```python
from build123d import *

# Parameters (mm, degrees)
SKETCH1_W              = 116
SKETCH1_H              = 60
SKETCH1_R              = 2
BOSS_EXTRUDE1_DEPTH    = 3
SKETCH2_R              = 1.75
ODROID_HOLES_DEPTH     = 4
CUT_EXTRUDE2_DEPTH     = 0.2
SKETCH4_R              = 1.75
PIXHAWK_PM_DEPTH       = 4
SKETCH5_R              = 1.75
BUCKCONVERTER_5A_DEPTH = 4
SKETCH6_R              = 2.5
SKETCH6_R_2            = 4.5
CUT_EXTRUDE5_DEPTH     = 4
FILLET1_R              = 5


with BuildPart() as part:
    # Sketch1 → Boss-Extrude1 (new body)
    with BuildSketch(Plane(origin=(0, 0, 0), x_dir=(1, 0, 0), z_dir=(0, 1, 0))):
        Rectangle(SKETCH1_W, SKETCH1_H)
        with Locations((53, 13)):
            Circle(SKETCH1_R, mode=Mode.SUBTRACT)
        with Locations((53, -13)):
            Circle(SKETCH1_R, mode=Mode.SUBTRACT)
        with Locations((-53, -13)):
            Circle(SKETCH1_R, mode=Mode.SUBTRACT)
        with Locations((-53, 13)):
            Circle(SKETCH1_R, mode=Mode.SUBTRACT)
    extrude(amount=BOSS_EXTRUDE1_DEPTH)

    # Sketch2 → Odroid-holes (cut, through all)
    with BuildSketch(Plane(origin=(0, 3, 0), x_dir=(1, 0, 0), z_dir=(0, 1, 0))):
        with Locations((38, 26)):
            Circle(SKETCH2_R)
        with Locations((38, -26)):
            Circle(SKETCH2_R)
        with Locations((-38, -26)):
            Circle(SKETCH2_R)
        with Locations((-38, 26)):
            Circle(SKETCH2_R)
    extrude(amount=-ODROID_HOLES_DEPTH, mode=Mode.SUBTRACT)

    # Sketch3 → Cut-Extrude2 (cut)
    with BuildSketch(Plane(origin=(0, 3, 0), x_dir=(1, 0, 0), z_dir=(0, 1, 0))):
        Polygon((-49.756039442, -1.122419343), (-49.756039442, -1.666214416), (-51.913411237, -0.552547549), (-51.913411237, -0.104155121), (-49.756039442, 1.009511746), (-49.756039442, 0.465080657), (-51.293930067, -0.328669343), align=None)
        Polygon((-47.110206109, -1.122419343), (-47.110206109, -1.666214416), (-49.267577904, -0.552547549), (-49.267577904, -0.104155121), (-47.110206109, 1.009511746), (-47.110206109, 0.465080657), (-48.648096734, -0.328669343), align=None)
        Polygon((-44.464372776, -1.122419343), (-44.464372776, -1.666214416), (-46.621744571, -0.552547549), (-46.621744571, -0.104155121), (-44.464372776, 1.009511746), (-44.464372776, 0.465080657), (-46.002263401, -0.328669343), align=None)
    extrude(amount=-CUT_EXTRUDE2_DEPTH, mode=Mode.SUBTRACT)

    # Sketch4 → Pixhawk-PM (cut, through all)
    with BuildSketch(Plane(origin=(0, 3, 0), x_dir=(1, 0, 0), z_dir=(0, 1, 0))):
        with Locations((-1, 15)):
            Circle(SKETCH4_R)
        with Locations((29, 15)):
            Circle(SKETCH4_R)
        with Locations((29, -15)):
            Circle(SKETCH4_R)
        with Locations((-1, -15)):
            Circle(SKETCH4_R)
    extrude(amount=-PIXHAWK_PM_DEPTH, mode=Mode.SUBTRACT)

    # Sketch5 → BuckConverter-5A (cut, through all)
    with BuildSketch(Plane(origin=(0, 3, 0), x_dir=(1, 0, 0), z_dir=(0, 1, 0))):
        with Locations((-9.1, 6.875)):
            Circle(SKETCH5_R)
        with Locations((-24.9, 6.875)):
            Circle(SKETCH5_R)
        with Locations((-24.9, -6.875)):
            Circle(SKETCH5_R)
        with Locations((-9.1, -6.875)):
            Circle(SKETCH5_R)
    extrude(amount=-BUCKCONVERTER_5A_DEPTH, mode=Mode.SUBTRACT)

    # Sketch6 → Cut-Extrude5 (cut, through all)
    with BuildSketch(Plane(origin=(0, 3, 0), x_dir=(1, 0, 0), z_dir=(0, 1, 0))):
        with Locations((37, 18)):
            Circle(SKETCH6_R)
        with Locations((37, -18)):
            Circle(SKETCH6_R)
        with Locations((-17, 0)):
            Circle(SKETCH6_R_2)
        with BuildLine():
            Line((-30, 23.75), (30, 23.75))
            ThreePointArc((30, 23.75), (31.75, 22), (30, 20.25))
            Line((30, 20.25), (-30, 20.25))
            ThreePointArc((-30, 20.25), (-31.75, 22), (-30, 23.75))
        make_face()
        with BuildLine():
            Line((-30, -23.75), (30, -23.75))
            ThreePointArc((30, -23.75), (31.75, -22), (30, -20.25))
            Line((30, -20.25), (-30, -20.25))
            ThreePointArc((-30, -20.25), (-31.75, -22), (-30, -23.75))
        make_face()
        with BuildLine():
            Line((-37, 15.75), (-17, 15.75))
            ThreePointArc((-17, 15.75), (-15.25, 14), (-17, 12.25))
            Line((-17, 12.25), (-37, 12.25))
            ThreePointArc((-37, 12.25), (-38.75, 14), (-37, 15.75))
        make_face()
        with BuildLine():
            Line((-37, -15.75), (-17, -15.75))
            ThreePointArc((-17, -15.75), (-15.25, -14), (-17, -12.25))
            Line((-17, -12.25), (-37, -12.25))
            ThreePointArc((-37, -12.25), (-38.75, -14), (-37, -15.75))
        make_face()
        with BuildLine():
            Line((-1.5, 10), (35.5, 10))
            ThreePointArc((35.5, 10), (36.914213562, 9.414213562), (37.5, 8))
            Line((37.5, 8), (37.5, -8))
            ThreePointArc((37.5, -8), (36.914213562, -9.414213562), (35.5, -10))
            Line((35.5, -10), (-1.5, -10))
            ThreePointArc((-1.5, -10), (-2.914213562, -9.414213562), (-3.5, -8))
            Line((-3.5, -8), (-3.5, 8))
            ThreePointArc((-3.5, 8), (-2.914213562, 9.414213562), (-1.5, 10))
        make_face()
        with BuildLine():
            Line((-31, 6), (-31, -6))
            ThreePointArc((-31, -6), (-34, -9), (-37, -6))
            Line((-37, -6), (-37, 6))
            ThreePointArc((-37, 6), (-34, 9), (-31, 6))
        make_face()
    extrude(amount=-CUT_EXTRUDE5_DEPTH, mode=Mode.SUBTRACT)

    # Fillet1
    fillet1_edges = [part.edges().sort_by_distance(p)[0] for p in [
        (58, 1.5, 30),
        (-58, 1.5, 30),
        (-58, 1.5, -30),
        (58, 1.5, -30),
    ]]
    fillet(fillet1_edges, radius=FILLET1_R)


solid = part.part
```
The listing builds one solid part. Answer for the finished solid, in the listing's coordinates (mm). A direction names the side the tool comes from. Coordinates: 2 decimals unless noted, no trailing zeros. Loops run counter-clockwise (first coordinate to the right, second up) from the corner with the lowest first, then second, coordinate; pieces in that order, holes last. Notation, with made-up numbers: M 21.5,81 L 27.5,81 A9 ccw 27.5,85 Z; hole C -4,-8.75 d3. An arc over 180 degrees is marked long. Answer as a JSON object with one key per item and string values. Group by question number.
Item 1: Which of the six approach directions +Z, -Z, +X, -X, +Y, -Y give full straight-line access (tool end or side, diameter ignored) to faces 4 (the face through (-51, 2.8, 0)), 5 (the face through (-1, 1, 30)), 6 (the face through (-2.9, 1.52, 9.43))?
Item 2: Consider L1, parallel to Z at x = -53, y = 1.4; L2, parallel to Z at x = -17, y = 1; L3, parallel to Z at x = 18, y = 2.7. Determine where each line is inside the solid, lowest interval first.
Item 3: This flat-tipped pin is pushed along its axis until it touches: P1, Ø4.5, axis at x = 38, z = 26, coming from the -Y side. Where does it stop, or does it pass through?
Item 4: Section A-A (x = -34) is taken. Write down the section's boundary in (y, z).
Item 5: Section B-B (y = 2) is taken. Give the number of separate pieces and of enclosed holes in the cut face, and give its area (3 significant figures).
Item 6: Determine the mould class of faces 1 (the face through (-37, 2, 0)), 2 (the face through (-1, 3, 13)), 3 (the face through (0, 2, 23.75)) for opening direction X: +X half, -X half, draft (parallel to the pull), parting line (faces both ways), or undercut.
Solved:
{
 "1": {"face 4": "+Y", "face 5": "+Z, +X, -X, +Y, -Y", "face 6": "+Y, -Y"},
 "2": {"L1": "z = -30 to -15, -11 to 11, 15 to 30", "L2": "z = -30 to -23.75, -20.25 to -15.75, -12.25 to -4.5, 4.5 to 12.25, 15.75 to 20.25, 23.75 to 30", "L3": "z = -30 to -23.75, -20.25 to -10, 10 to 20.25, 23.75 to 30"},
 "3": {"P1": "stops at y = 0"},
 "4": {"outline": "M 0,-30 L 3,-30 L 3,-15.75 L 0,-15.75 Z; M 0,-12.25 L 3,-12.25 L 3,-9 L 0,-9 Z; M 0,9 L 3,9 L 3,12.25 L 0,12.25 Z; M 0,15.75 L 3,15.75 L 3,30 L 0,30 Z"},
 "5": {"separate pieces": "1", "enclosed holes": "25", "area": "5,150 mm2"},
 "6": {"face 1": "undercut", "face 2": "draft", "face 3": "undercut"}
}
